Design review of the part built by this model. Coordinates are the model's own, in mm. Coordinates: 2 decimals unless noted, no trailing zeros. Write each loop counter-clockwise with the first axis right and the second up, starting at its lowest first coordinate (ties: lowest second). Pieces come first, ordered by that corner, then holes.
Q1. Take a section at A-A, the plane x = -24. Write out the cut boundary in (y, z).
Q2. Take a section at B-B, the plane z = 0.35. State how many separate pieces and enclosed holes the cut face has, plus the area to 3 significant figures.
Q3. For L1, parallel to X at y = -43, z = 1.6; L2, parallel to Y at x = 102, z = 0.4; L3, parallel to Y at x = -36, z = 1.55, list the stretches that pass through material, from the lowest coordinate up.
Q4. The part is to be moulded in two halves that separate along X. For faces 1 (the cylindrical face through (-37.683, -4.912, 1.014)), 2 (the flat face through (-2, 1, 0)), 3 (the flat face through (-111, 56, 1)), say which applies: released by +X, released by -X, zero draft, split by the parting line, or undercut.
Q5. For pin 1 Ø2.5 at (x, y) = (-41.23, -57) entering from +Z; pin 2 Ø6.5 at (x, y) = (-35.685, -5) entering from -Z; pin 3 Ø0.6 at (y, z) = (-57, 1) entering from -X, all flat-tipped, find the tip position at first contact; note any pin that passes through.
from build123d import *

# Parameters (mm, degrees)
SKETCH_5_W           = 230
SKETCH_5_H           = 120
EXTRUDE_2_DEPTH      = 2
SKETCH_6_R           = 2.5
CUT_EXTRUDE_3_DEPTH  = 130.726635661
SKETCH_7_R           = 1.5
SKETCH_7_W           = 6
SKETCH_7_H           = 6
CUT_EXTRUDE_4_DEPTH  = 130.726635661
SKETCH_8_R           = 1.5
SKETCH_8_W           = 6
SKETCH_8_H           = 6
CUT_EXTRUDE_5_DEPTH  = 130.726635661
SKETCH_9_R           = 2
SKETCH_9_W           = 40.7
SKETCH_9_H           = 20
CUT_EXTRUDE_6_DEPTH  = 130.726635661
SKETCH_10_R          = 1.3
CUT_EXTRUDE_7_DEPTH  = 130.726635661
SKETCH_11_R          = 1.3
CUT_EXTRUDE_8_DEPTH  = 130.726635661
SKETCH_12_R          = 1.9
CUT_EXTRUDE_9_DEPTH  = 130.726635661
SKETCH_13_W          = 3.8
SKETCH_13_H          = 20
CUT_EXTRUDE_10_DEPTH = 130.726635661
SKETCH_14_R          = 1.9
CUT_EXTRUDE_11_DEPTH = 130.726635661
SKETCH_17_R          = 3
CUT_EXTRUDE_12_DEPTH = 130.726635661
CHAMFER_1_SIZE       = 8


with BuildPart() as part:
    # 草图5 → 凸台-拉伸2 (new body)
    with BuildSketch(Plane.XY):
        Rectangle(SKETCH_5_W, SKETCH_5_H)
    extrude(amount=EXTRUDE_2_DEPTH)

    # 草图6 → 切除-拉伸3 (cut, through all)
    with BuildSketch(Plane.XY.offset(2)):
        with Locations((-24, 0)):
            Circle(SKETCH_6_R)
        with Locations((19.5, 25.11473671)):
            Circle(SKETCH_6_R)
        with Locations((19.5, -25.11473671)):
            Circle(SKETCH_6_R)
    extrude(amount=-CUT_EXTRUDE_3_DEPTH, mode=Mode.SUBTRACT)

    # 草图7 → 切除-拉伸4 (cut, through all)
    with BuildSketch(Plane.XY.offset(2)):
        with Locations((74, 57)):
            Circle(SKETCH_7_R)
        with Locations(Location((102, 57, 0), (0, 0, 180))):
            Circle(SKETCH_7_R)
        with Locations((102, -57)):
            Circle(SKETCH_7_R)
        with Locations(Location((74, -57, 0), (0, 0, 180))):
            Circle(SKETCH_7_R)
        with Locations((88, 57)):
            Rectangle(SKETCH_7_W, SKETCH_7_H)
        with Locations((88, -57)):
            Rectangle(SKETCH_7_W, SKETCH_7_H)
    extrude(amount=-CUT_EXTRUDE_4_DEPTH, mode=Mode.SUBTRACT)

    # 草图8 → 切除-拉伸5 (cut, through all)
    with BuildSketch(Plane.XY.offset(2)):
        with Locations((36.22, 28)):
            Circle(SKETCH_8_R)
        with Locations(Location((65.22, 28, 0), (0, 0, 180))):
            Circle(SKETCH_8_R)
        with Locations((65.22, -28)):
            Circle(SKETCH_8_R)
        with Locations(Location((36.22, -28, 0), (0, 0, 180))):
            Circle(SKETCH_8_R)
        with Locations((50.72, 28)):
            Rectangle(SKETCH_8_W, SKETCH_8_H)
        with Locations((50.72, -28)):
            Rectangle(SKETCH_8_W, SKETCH_8_H)
    extrude(amount=-CUT_EXTRUDE_5_DEPTH, mode=Mode.SUBTRACT)

    # 草图9 → 切除-拉伸6 (cut, through all)
    with BuildSketch(Plane.XY.offset(2)):
        with Locations((-84.315, 5)):
            Circle(SKETCH_9_R)
        with Locations(Location((-84.315, -5, 0), (0, 0, 180))):
            Circle(SKETCH_9_R)
        with Locations((-35.685, -5)):
            Circle(SKETCH_9_R)
        with Locations(Location((-35.685, 5, 0), (0, 0, 180))):
            Circle(SKETCH_9_R)
        with Locations((-60, 0)):
            Rectangle(SKETCH_9_W, SKETCH_9_H)
    extrude(amount=-CUT_EXTRUDE_6_DEPTH, mode=Mode.SUBTRACT)

    # 草图10 → 切除-拉伸7 (cut, through all)
    with BuildSketch(Plane.XY.offset(2)):
        with Locations((-41.227442559, 57)):
            Circle(SKETCH_10_R)
        with Locations(Location((-41.227442559, -57, 0), (0, 0, 180))):
            Circle(SKETCH_10_R)
        with Locations((-71.227442559, 57)):
            Circle(SKETCH_10_R)
        with Locations(Location((-71.227442559, -57, 0), (0, 0, 180))):
            Circle(SKETCH_10_R)
    extrude(amount=-CUT_EXTRUDE_7_DEPTH, mode=Mode.SUBTRACT)

    # 草图11 → 切除-拉伸8 (cut, through all)
    with BuildSketch(Plane.XY.offset(2)):
        with Locations((-100, 57)):
            Circle(SKETCH_11_R)
        with Locations((-80, 57)):
            Circle(SKETCH_11_R)
        with Locations(Location((-80, -57, 0), (0, 0, 180))):
            Circle(SKETCH_11_R)
        with Locations(Location((-100, -57, 0), (0, 0, 180))):
            Circle(SKETCH_11_R)
    extrude(amount=-CUT_EXTRUDE_8_DEPTH, mode=Mode.SUBTRACT)

    # 草图12 → 切除-拉伸9 (cut, through all)
    with BuildSketch(Plane.XY.offset(2)):
        with Locations((-48.073915411, 27)):
            Circle(SKETCH_12_R)
        with Locations(Location((-54.014113812, -43, 0), (0, 0, 180))):
            Circle(SKETCH_12_R)
        with Locations((-68.073915411, 27)):
            Circle(SKETCH_12_R)
        with Locations((-74.014113812, 43)):
            Circle(SKETCH_12_R)
        with Locations((-88.073915411, 27)):
            Circle(SKETCH_12_R)
        with Locations((-54.014113812, 43)):
            Circle(SKETCH_12_R)
        with Locations(Location((-88.073915411, -27, 0), (0, 0, 180))):
            Circle(SKETCH_12_R)
        with Locations(Location((-74.014113812, -43, 0), (0, 0, 180))):
            Circle(SKETCH_12_R)
        with Locations(Location((-68.073915411, -27, 0), (0, 0, 180))):
            Circle(SKETCH_12_R)
        with Locations(Location((-48.073915411, -27, 0), (0, 0, 180))):
            Circle(SKETCH_12_R)
    extrude(amount=-CUT_EXTRUDE_9_DEPTH, mode=Mode.SUBTRACT)

    # 草图13 → 切除-拉伸10 (cut, through all)
    with BuildSketch(Plane.XY.offset(2)):
        with Locations((-95, 0)):
            Rectangle(SKETCH_13_W, SKETCH_13_H)
        with Locations((-105, 0)):
            Rectangle(SKETCH_13_W, SKETCH_13_H)
    extrude(amount=-CUT_EXTRUDE_10_DEPTH, mode=Mode.SUBTRACT)

    # 草图14 → 切除-拉伸11 (cut, through all)
    with BuildSketch(Plane.XY.offset(2)):
        with Locations((-96.644922827, 33.589628644)):
            Circle(SKETCH_14_R)
        with Locations(Location((-96.644922827, -33.589628644, 0), (0, 0, 180))):
            Circle(SKETCH_14_R)
    extrude(amount=-CUT_EXTRUDE_11_DEPTH, mode=Mode.SUBTRACT)

    # 草图17 → 切除-拉伸12 (cut, through all)
    with BuildSketch(Plane.XY.offset(2)):
        with Locations((-77.855262933, 19.238416103)):
            Circle(SKETCH_17_R)
        with Locations(Location((-77.855262933, -19.238416103, 0), (0, 0, 180))):
            Circle(SKETCH_17_R)
    extrude(amount=-CUT_EXTRUDE_12_DEPTH, mode=Mode.SUBTRACT)

    # 倒角1
    chamfer_1_edges = [part.edges().sort_by_distance(p)[0] for p in [
        (-115, -60, 1),
        (-115, 60, 1),
    ]]
    chamfer(chamfer_1_edges, length=CHAMFER_1_SIZE)


solid = part.part
Responses:
1. outline: (-60, 0) - (-2.5, 0) - (-2.5, 2) - (-60, 2) - close; (2.5, 0) - (60, 0) - (60, 2) - (2.5, 2) - close
2. separate pieces: 1
2. enclosed holes: 42
2. area: 26,000 mm2
3. L1: x = -115 to -75.91, -72.11 to -55.91, -52.11 to 115
3. L2: y = -60 to -58.5, -55.5 to 55.5, 58.5 to 60
3. L3: y = -60 to -6.98, -3.02 to 3.02, 6.98 to 60
4. face 1: undercut
4. face 2: zero draft
4. face 3: released by -X
5. pin 1: passes through
5. pin 2: stops at z = 0
5. pin 3: stops at x = -110.3
